Could you check a few things on this model? Use its own coordinates, in mm. A direction names the side the tool comes from. Give positions to 0.01 mm unless a question says otherwise; leave off trailing zeros. Order: outer loops, then holes, each group sorted by start corner. A loop starts at its lowest first (then second) coordinate and runs counter-clockwise, first axis right, second up.
(1) Will these pins go through, and if not, where does the flat tip stop? pin 1 (2 mm diameter, centred on x = 507.5, z = 13, fed in from +Y); pin 2 (3 mm diameter, centred on x = -135, y = -10.5, fed in from -Z); pin 3 (8 mm diameter, centred on y = -20, z = 221, fed in from +X).
(2) Imagine slicing it at A-A, the plane z = -130.5. Write out the boundary of the cut face in (x, y), then the cut area to 3 significant figures.
(3) Imagine slicing it at B-B, the plane x = -380. Write out the boundary of the cut face in (y, z).
(4) If we mould it in two halves opening along X, with no side actions, what happens to faces 4 (the flat face through (-755, -2, -2)), 5 (the flat face through (650, -24, 225)), 6 (the flat face through (227.5, -26, -7))? For each: released by +X, released by -X, zero draft, split by the parting line, or undercut.
(5) If I drill on probe 1 along Z at (x, y) = (205, -6); probe 2 along Z at (x, y) = (-440.5, 2.5); probe 3 along X at (y, z) = (2, 233), over which ranges is the centre line in solid material (lowest first)?
(6) On a 3-axis mill with a long thin cutter (end or side, diameter ignored), from which of +Z, -Z, +X, -X, +Y, -Y can I reach the whole of each face in a straight line? I mean faces 1 (the flat face through (-11, -5, 324)), 2 (the flat face through (-10, 0, -6)), 3 (the flat face through (252.5, -26, -7)). Say none if no direction works.
from build123d import *

# Parameters (mm, degrees)
SKETCH2_W                 = 1510
SKETCH2_H                 = 810
SKETCH2_W_2               = 1500
SKETCH2_H_2               = 800
BOSS_EXTRUDE1_DEPTH       = 10
SKETCH3_W                 = 1510
SKETCH3_H                 = 810
SKETCH3_W_2               = 1460
SKETCH3_H_2               = 140
SKETCH3_W_3               = 30
SKETCH3_H_3               = 400
SKETCH3_W_4               = 1200
BOSS_EXTRUDE2_DEPTH       = 5
SKETCH5_W                 = 1510
SKETCH5_H                 = 5
BOSS_EXTRUDE3_DEPTH       = 10
LPATTERN1_COUNT           = 2
LPATTERN1_PITCH           = 35
LPATTERN2_COUNT           = 2
LPATTERN2_PITCH           = 440
LPATTERN2_COPY_1_SKETCH_W = 1510
LPATTERN2_COPY_1_SKETCH_H = 5
LPATTERN2_COPY_1_DEPTH    = 10
SKETCH6_R                 = 10
BOSS_EXTRUDE4_DEPTH       = 5
LPATTERN3_COUNT           = 2
LPATTERN3_PITCH           = 440
SKETCH8_R                 = 10
BOSS_EXTRUDE5_DEPTH       = 25
SKETCH9_W                 = 80
SKETCH9_H                 = 400
BOSS_EXTRUDE6_DEPTH       = 5
SKETCH10_R                = 10
BOSS_EXTRUDE7_DEPTH       = 12.5
SKETCH12_W                = 400
SKETCH12_H                = 5
BOSS_EXTRUDE8_DEPTH       = 100
FILLET3_R                 = 10
FILLET4_R                 = 10
FILLET5_R                 = 10
FILLET6_R                 = 10
SKETCH13_W                = 1460
SKETCH13_H                = 140
SKETCH13_W_2              = 800
SKETCH13_H_2              = 400
SKETCH13_W_3              = 30
SKETCH13_W_4              = 220
BOSS_EXTRUDE9_DEPTH       = 5


with BuildPart() as part:
    # Sketch2 → Boss-Extrude1 (new body)
    with BuildSketch(Plane(origin=(0, 0, 0), x_dir=(1, 0, 0), z_dir=(0, 1, 0))):
        Rectangle(SKETCH2_W, SKETCH2_H)
        Rectangle(SKETCH2_W_2, SKETCH2_H_2, mode=Mode.SUBTRACT)
    extrude(amount=BOSS_EXTRUDE1_DEPTH)

    # Sketch3 → Boss-Extrude2 (add)
    with BuildSketch(Plane(origin=(0, 0, 0), x_dir=(1, 0, 0), z_dir=(0, 1, 0))):
        Rectangle(SKETCH3_W, SKETCH3_H)
        with Locations((0, -310)):
            Rectangle(SKETCH3_W_2, SKETCH3_H_2, mode=Mode.SUBTRACT)
        with Locations((0, 310)):
            Rectangle(SKETCH3_W_2, SKETCH3_H_2, mode=Mode.SUBTRACT)
        with Locations((-715, 0)):
            Rectangle(SKETCH3_W_3, SKETCH3_H_3, mode=Mode.SUBTRACT)
        with Locations((715, 0)):
            Rectangle(SKETCH3_W_3, SKETCH3_H_3, mode=Mode.SUBTRACT)
        Rectangle(SKETCH3_W_4, SKETCH3_H_3, mode=Mode.SUBTRACT)
    extrude(amount=-BOSS_EXTRUDE2_DEPTH)

    # Sketch5 → Boss-Extrude3 (add)
    with BuildSketch(Plane.XZ.offset(5)):
        with Locations((0, 237.5)):
            Rectangle(SKETCH5_W, SKETCH5_H)
    boss_extrude3 = extrude(amount=BOSS_EXTRUDE3_DEPTH)

    # LPattern1: Boss-Extrude3 ×2
    with Locations(*[(0, 0, -i * LPATTERN1_PITCH) for i in range(1, LPATTERN1_COUNT)]):
        add(boss_extrude3)

    # LPattern2: Boss-Extrude3 ×2
    with Locations(*[(0, 0, -i * LPATTERN2_PITCH) for i in range(1, LPATTERN2_COUNT)]):
        add(boss_extrude3)

    # LPattern2 copy 1 sketch → LPattern2 copy 1 (add)
    with BuildSketch(Plane(origin=(0, -5, -475), x_dir=(1, 0, 0), z_dir=(0, -1, 0))):
        with Locations((0, 237.5)):
            Rectangle(LPATTERN2_COPY_1_SKETCH_W, LPATTERN2_COPY_1_SKETCH_H)
    extrude(amount=LPATTERN2_COPY_1_DEPTH)

    # Sketch6 → Boss-Extrude4 (add, symmetric)
    with BuildSketch(Plane.XY.offset(220)):
        with BuildLine():
            Line((630, -5), (630, -35))
            ThreePointArc((630, -35), (650, -55), (670, -35))
            Line((670, -35), (670, -5))
            Line((670, -5), (630, -5))
        make_face()
        with Locations((650, -35)):
            Circle(SKETCH6_R, mode=Mode.SUBTRACT)
    boss_extrude4 = extrude(amount=BOSS_EXTRUDE4_DEPTH, both=True)

    # LPattern3: Boss-Extrude4 ×2
    with Locations(*[(0, 0, -i * LPATTERN3_PITCH) for i in range(1, LPATTERN3_COUNT)]):
        add(boss_extrude4)

    # Sketch8 → Boss-Extrude5 (add)
    with BuildSketch(Plane.ZY.offset(755)):
        with BuildLine():
            Line((-25, -35), (-25, -5))
            Line((-25, -5), (25, -5))
            Line((25, -5), (25, -35))
            ThreePointArc((25, -35), (0, -60), (-25, -35))
        make_face()
        with Locations((0, -35)):
            Circle(SKETCH8_R, mode=Mode.SUBTRACT)
    extrude(amount=-BOSS_EXTRUDE5_DEPTH)

    # Sketch9 → Boss-Extrude6 (add)
    with BuildSketch(Plane(origin=(0, 0, 0), x_dir=(1, 0, 0), z_dir=(0, 1, 0))):
        with Locations((240, 0)):
            Rectangle(SKETCH9_W, SKETCH9_H)
    extrude(amount=-BOSS_EXTRUDE6_DEPTH)

    # Sketch10 → Boss-Extrude7 (add, symmetric)
    with BuildSketch(Plane.ZY.offset(-240)):
        with BuildLine():
            Line((25, -5), (25, -35))
            ThreePointArc((25, -35), (0, -60), (-25, -35))
            Line((-25, -35), (-25, -5))
            Line((-25, -5), (25, -5))
        make_face()
        with Locations((0, -35)):
            Circle(SKETCH10_R, mode=Mode.SUBTRACT)
    extrude(amount=BOSS_EXTRUDE7_DEPTH, both=True)

    # Sketch12 → Boss-Extrude8 (add)
    with BuildSketch(Plane(origin=(280, 0, 0), x_dir=(0, 0, -1), z_dir=(1, 0, 0))):
        with Locations((0, -2.5)):
            Rectangle(SKETCH12_W, SKETCH12_H)
    extrude(amount=BOSS_EXTRUDE8_DEPTH)

    # Fillet3
    fillet3_edges = [part.edges().sort_by_distance(p)[0] for p in [
        (240, -5, 25),
    ]]
    fillet(fillet3_edges, radius=FILLET3_R)

    # Fillet4
    fillet4_edges = [part.edges().sort_by_distance(p)[0] for p in [
        (240, -5, -25),
    ]]
    fillet(fillet4_edges, radius=FILLET4_R)

    # Fillet5
    fillet5_edges = [part.edges().sort_by_distance(p)[0] for p in [
        (-742.5, -5, 25),
    ]]
    fillet(fillet5_edges, radius=FILLET5_R)

    # Fillet6
    fillet6_edges = [part.edges().sort_by_distance(p)[0] for p in [
        (-742.5, -5, -25),
    ]]
    fillet(fillet6_edges, radius=FILLET6_R)

    # Sketch13 → Boss-Extrude9 (add)
    with BuildSketch(Plane.XZ.offset(5)):
        with Locations((0, 310)):
            Rectangle(SKETCH13_W, SKETCH13_H)
        with Locations((0, -310)):
            Rectangle(SKETCH13_W, SKETCH13_H)
        with Locations((-200, 0)):
            Rectangle(SKETCH13_W_2, SKETCH13_H_2)
        with Locations((-715, 0)):
            Rectangle(SKETCH13_W_3, SKETCH13_H_2)
        with Locations((490, 0)):
            Rectangle(SKETCH13_W_4, SKETCH13_H_2)
        with Locations((715, 0)):
            Rectangle(SKETCH13_W_3, SKETCH13_H_2)
    extrude(amount=-BOSS_EXTRUDE9_DEPTH)


solid = part.part
Answer block:
1. pin 1: stops at y = 0
1. pin 2: stops at z = -240
1. pin 3: stops at x = 670
2. outline: (-755, -5) - (755, -5) - (755, 10) - (750, 10) - (750, 0) - (-750, 0) - (-750, 10) - (-755, 10) - close
2. area: 7,650 mm2
3. outline: (-15, -240) - (-5, -240) - (-5, -405) - (10, -405) - (10, -400) - (0, -400) - (0, 400) - (10, 400) - (10, 405) - (-5, 405) - (-5, 240) - (-15, 240) - (-15, 235) - (-5, 235) - (-5, 205) - (-15, 205) - (-15, 200) - (-5, 200) - (-5, -200) - (-15, -200) - (-15, -205) - (-5, -205) - (-5, -235) - (-15, -235) - close
4. face 4: released by -X
4. face 5: zero draft
4. face 6: undercut
5. probe 1: z = -240 to -235, -205 to -200, 200 to 205, 235 to 240
5. probe 2: z = -405 to -400, 400 to 405
5. probe 3: x = -755 to -750, 750 to 755
6. face 1: +Z, +X, -X, -Y
6. face 2: +Y
6. face 3: +X, -Y
